```python
from build123d import *

# Parameters (mm, degrees)
BOSS_EXTRUDE1_DEPTH = 2.5
FILLET1_R           = 10
SKETCH2_W           = 2.5
SKETCH2_H           = 30
BOSS_EXTRUDE2_DEPTH = 5
FILLET2_R           = 5
SKETCH3_R           = 15
SKETCH3_R_2         = 10
CUT_EXTRUDE1_DEPTH  = 5
FILLET3_R           = 30
FILLET4_R           = 5


# Some blends are built 0.0001 mm under size
with BuildPart() as part:
    # Sketch1 → Boss-Extrude1 (new, symmetric)
    with BuildSketch(Plane.XY):
        Polygon((-30.132236367, -289.114804685), (19.867763633, -317.982318144), (44.867763633, -317.982318144), (44.867763633, -217.982318144), (24.867763633, -217.982318144), (24.867763633, -287.982318144), (19.867763633, -287.982318144), (19.867763633, -72.512264306), (-134.182504853, -149.335156244), (-168.696300973, -209.114804685), (-157.870983425, -215.364804685), (-147.870983425, -198.044296609), (-143.540856406, -200.544296609), (-153.540856406, -217.864804685), (-142.715538859, -224.114804685), (-112.715538859, -172.153280458), (-58.588951122, -203.403280458), (-48.588951122, -186.082772382), (-44.258824104, -188.582772382), (-54.258824104, -205.903280458), (-0.132236367, -237.153280458), align=None)
    extrude(amount=BOSS_EXTRUDE1_DEPTH, both=True)

    # Fillet1
    fillet1_edges = [part.edges().sort_by_distance(p)[0] for p in [
        (-168.696300973, -209.114804685, 0),
        (-142.715538859, -224.114804685, 0),
        (-30.132236367, -289.114804685, 0),
        (19.867763633, -317.982318144, 0),
        (24.867763633, -217.982318144, 0),
        (44.867763633, -217.982318144, 0),
        (44.867763633, -317.982318144, 0),
    ]]
    fillet(fillet1_edges, radius=FILLET1_R - 0.0001)  # a hair under: the kernel refuses the full size

    # Sketch2 → Boss-Extrude2 (add)
    with BuildSketch(Plane.XY.offset(2.5)):
        with Locations((21.117763633, -87.512264306)):
            Rectangle(SKETCH2_W, SKETCH2_H)
    extrude(amount=-BOSS_EXTRUDE2_DEPTH)

    # Fillet2
    # the kernel refuses this fillet: 5 mm, written as the material it takes off along each edge
    with BuildSketch(Plane(origin=(22.367763633, -72.512264306, 13.325317547), x_dir=(-1, 0, 0), z_dir=(0, 0, -1))) as fillet2_piece_1:
        with BuildLine():
            CenterArc((5, -4.330127019), FILLET2_R, 120, 60)
            Line((0, -4.330127019), (-0.1, -4.330127019))
            Line((-0.1, -4.330127019), (-0.1, 0))
            Line((-0.1, 0), (0, 0.1))
            ThreePointArc((0, 0.1), (1.25, 0.1), (2.45, 0.08660254))
            Line((2.45, 0.08660254), (2.5, 0))
        make_face()
    extrude(amount=26.650635095, mode=Mode.SUBTRACT)

    # Sketch3 → Cut-Extrude1 (cut)
    with BuildSketch(Plane.XY.offset(2.5)):
        with Locations((-27.097618997, -153.858693218)):
            Circle(SKETCH3_R)
        with Locations((-6.775273551, -118.659358377)):
            Circle(SKETCH3_R_2)
    extrude(amount=-CUT_EXTRUDE1_DEPTH, mode=Mode.SUBTRACT)

    # Fillet3
    fillet3_edges = [part.edges().sort_by_distance(p)[0] for p in [
        (-134.182504853, -149.335156244, 0),
    ]]
    fillet(fillet3_edges, radius=FILLET3_R)

    # Fillet4
    fillet4_edges = [part.edges().sort_by_distance(p)[0] for p in [
        (-112.715538859, -172.153280458, 0),
        (-0.132236367, -237.153280458, 0),
    ]]
    fillet(fillet4_edges, radius=FILLET4_R)


solid = part.part
```
Check sheet for the modelled part. Datum: model origin and axes. Units: mm. A direction names the side the tool comes from. Coordinates: 2 decimals unless noted, no trailing zeros. Write each loop counter-clockwise with the first axis right and the second up, starting at its lowest first coordinate (ties: lowest second). Pieces come first, ordered by that corner, then holes. Notation, with made-up numbers: M 4.5,62.25 L 25.5,62.25 A14 ccw 25.5,70.25 Z; hole C 87,44.5 d8. An arc over 180 degrees is marked long. Use one line per item in the form item = value.
Item 1: Release check for a two-part mould opening along Y. For faces 5 (the face through (19.92, -317.63, 0.04)), 6 (the face through (-38, -194, -2.5)), 7 (the face through (2.763, -115.656, 0.035)) record: pulls with the +Y half, pulls with the -Y half, needs draft (parallel to the pull), parting line crosses it, or undercut.
Answer below:
face_5 = pulls with the -Y half
face_6 = needs draft
face_7 = undercut
Item 2: Sectioned sample at C-C, the plane z = 1.6. State how many separate pieces and enclosed holes the cut face has, and give its area (3 significant figures).
Answer below:
separate_pieces = 1
enclosed_holes = 2
area = 19,500 mm^2
Item 3: Sectioned sample at D-D, the plane x = -119. Record the cut outline in (y, z).
Answer below:
outline = M -183.04,-2.5 L -141.76,-2.5 L -141.76,2.5 L -183.04,2.5 Z
Item 4: Sectioned sample at B-B, the plane y = -112.5. Record the cut outline in (x, z).
Answer below:
outline = M -60.32,-2.5 L -14.65,-2.5 L -14.65,2.5 L -60.32,2.5 Z; M 1.1,-2.5 L 19.87,-2.5 L 19.87,2.5 L 1.1,2.5 Z
Item 5: Sectioned sample at A-A, the plane x = -29.5. Record the cut outline in (y, z).
Answer below:
outline = M -220.2,-2.5 L -168.67,-2.5 L -168.67,2.5 L -220.2,2.5 Z; M -139.05,-2.5 L -97.13,-2.5 L -97.13,2.5 L -139.05,2.5 Z
Item 6: Set-up check for faces 1 (the face through (22.368, -90, 0)), 2 (the face through (19.868, -197, 0)), 3 (the face through (-13.725, -260.696, 0.035)), 4 (the face through (24.868, -258, 0)): record each of +Z, -Z, +X, -X, +Y, -Y from which the full face is reachable in a straight line by a thin tool's end or side.
Answer below:
face_1 = +Z, -Z, +X, +Y
face_2 = +Z, -Z
face_3 = +Z, -Z, -X
face_4 = +Z, -Z, +Y
Item 7: Material ranges on L1, parallel to X at y = -212.5, z = -1.55; L2, parallel to X at y = -189.5, z = 0.9; L3, parallel to Y at x = -12, z = 0, recorded low to high. Write a range as from..to.
Answer below:
L1 = -162.13..-156.22, -150.44..-136.01, -42.83..19.87
L2 = -157.37..-122.73, -82.67..-50.56, -44.79..19.87
L3 = -299.58..-257.71, -230.3..-127.19, -110.13..-88.4
Item 8: Gauge pin test, flat ends, axial feed: pin 1 Ø2.5 at (y, z) = (-263, -0.5) entering from -X; pin 2 Ø0.8 at (x, z) = (21.5, -0.5) entering from -Y; pin 3 Ø1.5 at (x, z) = (-143.5, -1.5) entering from +Y. Record the tip position at first contact, or that the pin passes through.
Answer below:
pin_1 = -15.78
pin_2 = -317.96
pin_3 = -164.17
